Design review of the part shown in the three views and the two pictorial views. Dimensions are in mm from the part's minimum x, y and z. A direction names the side the tool comes from. Round coordinates to 2 decimals unless told otherwise and drop trailing zeros. Order: outer loops, then holes, each group sorted by start corner. A loop starts at its lowest first (then second) coordinate and runs counter-clockwise, first axis right, second up. Notation, with made-up numbers: M -26.75,44 L -22.75,44 A16 cw -22.75,72 Z; hole C -33,23.25 d9. An arc over 180 degrees is marked long. Use a Markdown table: item, result. Add a question column.
(1) To check wall thickness, follow probe 1 along Y at (x, z) = (5, 17.5); probe 2 along X at (y, z) = (5.25, 19.75); probe 3 along X at (y, z) = (5, 6). State the ranges of each line that lie inside material, in increasing order. Write a range as from..to.
(2) Take a section at B-B (z = 11). Write out the cut boundary in (x, y), then the cut area to 3 significant figures.
(3) Machinability: for the marked faces 5 and 6, which of the approach directions +Z, -Z, +X, -X, +Y, -Y give a long, thin tool a straight path to every point of the face, cutting with its end or side? Answer none if there is none.
(4) For pin 1 (4 mm diameter, centred on x = 29, y = 19, fed in from -Z); pin 2 (9 mm diameter, centred on x = 16.95, z = 11, fed in from +Y); pin 3 (9 mm diameter, centred on x = 6, y = 11, fed in from -Z), all flat-tipped, find the tip position at first contact; note any pin that passes through.
(5) Take a section at C-C (x = 5). Write out the cut boundary in (y, z).
(6) Take a section at D-D (y = 26.5). Write out the cut boundary in (x, z), then the cut area to 3 significant figures.
(7) The part is to be moulded in two halves that separate along Z. For the marked faces 1, 2, 3 and 4, say which applies: released by +Z, released by -Z, zero draft, split by the parting line, or undercut.
(8) Take a section at A-A (y = 6). Write out the cut boundary in (x, z).
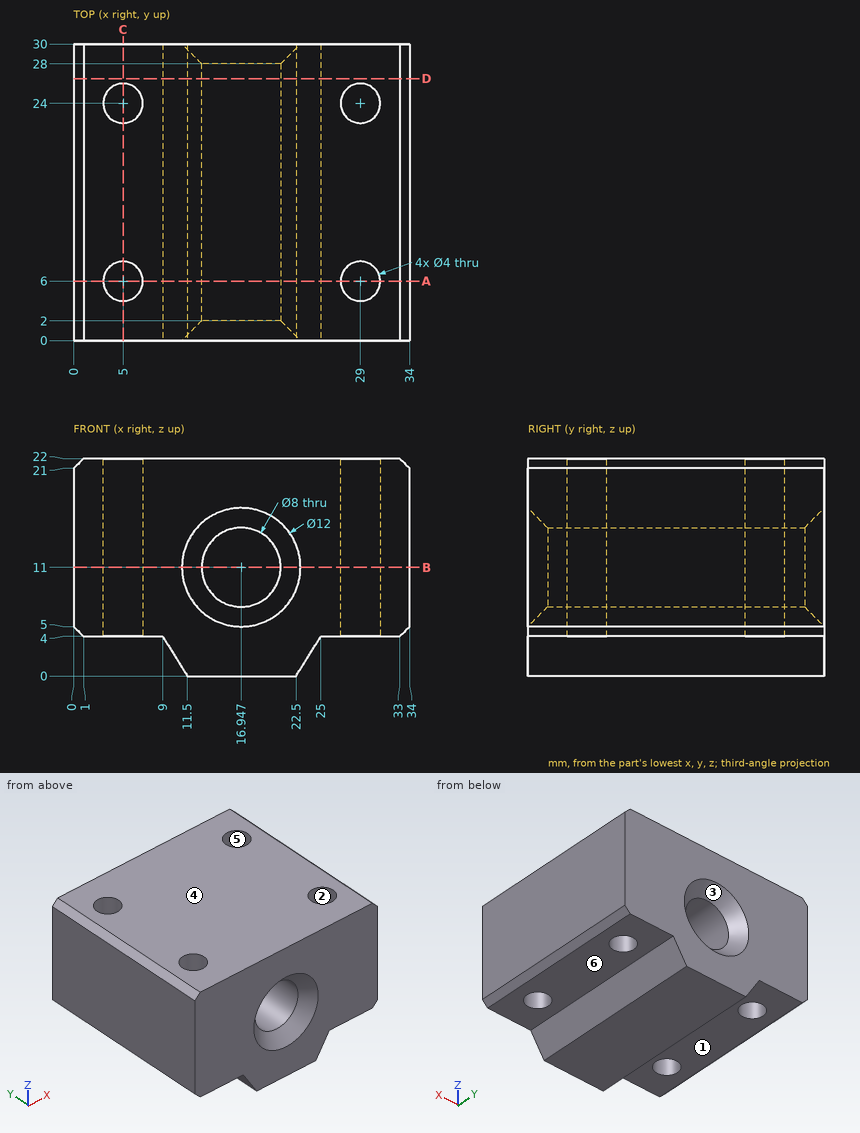
Verdict:
| question | item | result |
|---|---|---|
| 1 | probe 1 | y = 0..4, 8..22, 26..30 |
| 1 | probe 2 | x = 0..3.15, 6.85..27.15, 30.85..34 |
| 1 | probe 3 | x = 0..3.27, 6.73..27.27, 30.73..34 |
| 2 | outline | M 0,0 L 10.95,0 L 12.95,2 L 12.95,28 L 10.95,30 L 0,30 Z; M 20.95,2 L 22.95,0 L 34,0 L 34,30 L 22.95,30 L 20.95,28 Z; hole C 5,6 d4; hole C 5,24 d4; hole C 29,6 d4; hole C 29,24 d4 |
| 2 | area | 722 mm^2 |
| 3 | face 5 | +Z, -Z |
| 3 | face 6 | -Z, +X, +Y, -Y |
| 4 | pin 1 | stops at z = 4 |
| 4 | pin 2 | stops at y = 28.5 |
| 4 | pin 3 | stops at z = 1.6 |
| 5 | outline | M 0,4 L 4,4 L 4,22 L 0,22 Z; M 8,4 L 22,4 L 22,22 L 8,22 Z; M 26,4 L 30,4 L 30,22 L 26,22 Z |
| 6 | outline | M 0,5 L 1,4 L 9,4 L 11.5,0 L 22.5,0 L 25,4 L 33,4 L 34,5 L 34,21 L 33,22 L 1,22 L 0,21 Z; hole C 16.95,11 d8 |
| 6 | area | 614 mm^2 |
| 7 | face 1 | released by -Z |
| 7 | face 2 | zero draft |
| 7 | face 3 | undercut |
| 7 | face 4 | released by +Z |
| 8 | outline | M 0,5 L 1,4 L 3,4 L 3,22 L 1,22 L 0,21 Z; M 7,4 L 9,4 L 11.5,0 L 22.5,0 L 25,4 L 27,4 L 27,22 L 7,22 Z; M 31,4 L 33,4 L 34,5 L 34,21 L 33,22 L 31,22 Z; hole C 16.95,11 d8 |
